Could you check a few things on this model? Use its own coordinates, in mm. A direction names the side the tool comes from. Round coordinates to 2 decimals unless told otherwise and drop trailing zeros. Loops run counter-clockwise (first coordinate to the right, second up) from the corner with the lowest first, then second, coordinate; pieces in that order, holes last. Notation, with made-up numbers: M -9,18.5 L 47,18.5 A21 ccw 47,57.5 Z; hole C 61.25,82 d2. An arc over 180 degrees is marked long. One line per item, written item: value. Start each with the question number.
Q1. Imagine slicing it at D-D (y = 28). Please give me the cut outline in (x, z).
Q2. Please list where these lines run through material, in increasing order: line 1 along Y through (x, z) = (36.5, 12.5); line 2 along X through (y, z) = (20, 20.5); line 3 along X through (y, z) = (25.5, 13.5).
Q3. Imagine slicing it at A-A (z = 12). Please give me the cut outline in (x, y).
Q4. I'm going to push flat-ended pins straight in: pin 1 Ø9.5 at (x, z) = (31.5, 23.5) entering from +Y; pin 2 Ø6 at (y, z) = (30.5, 17) entering from +X. Where does each tip first touch, or does it pass through?
Q5. Imagine slicing it at C-C (z = 7.5). Please give me the cut outline in (x, y), then the cut area to 3 significant figures.
Q6. Imagine slicing it at B-B (x = 35). Please give me the cut outline in (y, z), then the cut area to 3 significant figures.
Q7. Which directions (+Z, -Z, +X, -X, +Y, -Y) give clear straight access to the entire face, cutting with the end or side of a thin tool? Please do faces 1 (the face through (53.84, 18.96, 16.1)), 2 (the face through (25.31, 6.26, 16.1)), 3 (the face through (25.49, 31.84, 15.65)).
from build123d import *

# Parameters (mm, degrees)
F1_DEPTH = 31.75
F3_DEPTH = 12.7
F5_DEPTH = 25.401
F7_DEPTH = 12.7


with BuildPart() as f1:
    # F0 (on Top) → F1 (new body)
    with BuildSketch(Plane.XY):
        Polygon((0, 38.1), (0, 0), (31.75, 0), (31.75, 12.7), (63.5, 12.7), (63.5, 25.4), (31.75, 25.4), (31.75, 38.1), align=None)
    extrude(amount=F1_DEPTH)

    # F2 (on face) → F3 (cut)
    with BuildSketch(Plane.XZ):
        Polygon((31.75, 31.75), (19.05, 31.75), (31.75, 0), align=None)
    extrude(amount=-F3_DEPTH, mode=Mode.SUBTRACT)

    # F4 (on face) → F5 (cut, through all)
    with BuildSketch(Plane.XZ.offset(-12.7)):
        Polygon((63.5, 31.75), (44.45, 31.75), (63.5, 0), align=None)
    extrude(amount=-F5_DEPTH, mode=Mode.SUBTRACT)

    # F6 (on face) → F7 (cut)
    with BuildSketch(Plane(origin=(0, 38.1, 0), x_dir=(-1, 0, 0), z_dir=(0, 1, 0))):
        Polygon((-31.75, 0), (-19.05, 31.75), (-31.75, 31.75), align=None)
    extrude(amount=-F7_DEPTH, mode=Mode.SUBTRACT)


solid = f1.part
Report:
1. outline: M 0,0 L 31.75,0 L 19.05,31.75 L 0,31.75 Z
2. line 1: y = 12.7 to 25.4
2. line 2: x = 0 to 51.2
2. line 3: x = 0 to 26.35
3. outline: M 0,0 L 26.95,0 L 26.95,12.7 L 56.3,12.7 L 56.3,25.4 L 26.95,25.4 L 26.95,38.1 L 0,38.1 Z
4. pin 1: stops at y = 25.4
4. pin 2: stops at x = 26.15
5. outline: M 0,0 L 28.75,0 L 28.75,12.7 L 59,12.7 L 59,25.4 L 28.75,25.4 L 28.75,38.1 L 0,38.1 Z
5. area: 1,480 mm²
6. outline: M 12.7,0 L 25.4,0 L 25.4,31.75 L 12.7,31.75 Z
6. area: 403 mm²
7. face 1: +Z, +X, +Y, -Y
7. face 2: +Z, +X, -Y
7. face 3: +Z, +X, +Y
